For this review, take the finished solid that the model builds, in its own axes (mm). A direction names the side the tool comes from. Give positions to 0.01 mm unless a question says otherwise; leave off trailing zeros. Write each loop counter-clockwise with the first axis right and the second up, starting at its lowest first coordinate (ties: lowest second). Pieces come first, ordered by that corner, then holes. Notation, with made-up numbers: M 85,-30.5 L 96,-30.5 A26 cw 96,-5.5 Z; hole C 85,2 d5. An arc over 180 degrees is marked long. Use one line per item in the form item = value. Start each with the question number.
Q1. Clearance check with flat-ended pins moving along their axes: pin 1 Ø1.8 at (y, z) = (5.5, 4) entering from +X; pin 2 Ø1.7 at (x, y) = (8, -3) entering from -Z; pin 3 Ø2.5 at (y, z) = (5, 8.5) entering from -X; pin 4 Ø4 at (x, z) = (0, 0) entering from -Y. State where each tip first meets the part, or that it passes through.
Q2. Consider section A-A on x = -82.55. Write out the cut boundary in (y, z).
Q3. Consider section C-C on x = -16. Write out the cut boundary in (y, z), and give its area (3 significant figures).
Q4. Tool access review of faces 1 (the flat face through (0, -3, -4.158)), 2 (the flat face through (-83, 4, 4.158)), 3 (the flat face through (-154, -16, 0.211)), 4 (the flat face through (-42, -3, -10)): name each direction out of +Z, -Z, +X, -X, +Y, -Y from which nothing blocks a thin tool from reaching the whole face with its end or side.
Q5. Mouldability with a two-part tool opening along Z and no side actions: class faces 5 (the cylindrical face through (-145.455, -23.522, -2.686)), 6 (the flat face through (-74, -6.35, 0)), 7 (the cylindrical face through (-85.967, -1.878, -0.759)) as released by +Z, released by -Z, zero draft, split by the parting line, or undercut.
Q6. For probe 1 along X at (y, z) = (-1, 0); probe 2 along X at (y, z) = (-2, -2.5); probe 3 along Y at (x, z) = (-106, 3.5), list the stretches that pass through material, from the lowest coordinate up. Write a range as [from, to].
Q7. Consider section B-B on y = -21.5. Write out the cut boundary in (x, z).
Q8. Consider section D-D on z = -6. Give the number of separate pieces and of enclosed holes in the cut face, and give its area (3 significant figures).
```python
from build123d import *

# Parameters (mm, degrees)
BOSS_EXTRUDE1_DEPTH   = 7.62
BOSS_EXTRUDE1_2_DEPTH = 7.62
BOSS_EXTRUDE1_3_DEPTH = 7.62
BOSS_EXTRUDE1_4_DEPTH = 7.62
SKETCH2_W             = 165.1
SKETCH2_H             = 20
BOSS_EXTRUDE2_DEPTH   = 6.35
LPATTERN2_COUNT       = 2
LPATTERN2_PITCH       = 82.55
CUT_EXTRUDE1_DEPTH    = 157.048617104
FILLET1_R             = 2.54
SKETCH13_R            = 3.5
CUT_EXTRUDE5_DEPTH    = 156.608722121
FILLET6_R             = 2.54
SKETCH14_W            = 8.89
SKETCH14_H            = 5.842
CUT_EXTRUDE6_DEPTH    = 157.048617104
SKETCH15_W            = 25.4
SKETCH15_H            = 40.894
BOSS_EXTRUDE3_DEPTH   = 12.7
FILLET15_R            = 10.16
FILLET16_R            = 10.16
FILLET17_R            = 10.16
FILLET18_R            = 10.16
SKETCH18_R            = 1.984375
CUT_EXTRUDE9_DEPTH    = 12.7


with BuildPart() as part:
    # Sketch1 → Boss-Extrude1 (new body)
    with BuildSketch(Plane(origin=(0, 0, 0), x_dir=(1, 0, 0), z_dir=(0, 1, 0))):
        Polygon((2.9718, 10), (-2.9718, 10), (-2.9718, 7.714), (-4.567901235, 7.714), (-4.567901235, 6.444), (-2.9718, 4.158), (2.9718, 4.158), (4.322098765, 6.444), (4.322098765, 7.714), (2.9718, 7.714), align=None)
    boss_extrude1 = extrude(amount=BOSS_EXTRUDE1_DEPTH)



with BuildPart() as body_2:
    # Sketch1 → Boss-Extrude1 2 (new body)
    with BuildSketch(Plane(origin=(0, 0, 0), x_dir=(1, 0, 0), z_dir=(0, 1, 0))):
        Polygon((4.158, -2.9718), (4.158, 2.9718), (6.444, 4.322098765), (7.714, 4.322098765), (7.714, 2.9718), (10, 2.9718), (10, -2.9718), (7.714, -2.9718), (7.714, -4.567901235), (6.444, -4.567901235), align=None)
    boss_extrude1_2 = extrude(amount=BOSS_EXTRUDE1_2_DEPTH)


with BuildPart() as body_3:
    # Sketch1 → Boss-Extrude1 3 (new body)
    with BuildSketch(Plane(origin=(0, 0, 0), x_dir=(1, 0, 0), z_dir=(0, 1, 0))):
        Polygon((-10, -2.9718), (-10, 2.9718), (-7.714, 2.9718), (-7.714, 4.567901235), (-6.444, 4.567901235), (-4.158, 2.9718), (-4.158, -2.9718), (-6.444, -4.322098765), (-7.714, -4.322098765), (-7.714, -2.9718), align=None)
    boss_extrude1_3 = extrude(amount=BOSS_EXTRUDE1_3_DEPTH)


with BuildPart() as body_4:
    # Sketch1 → Boss-Extrude1 4 (new body)
    with BuildSketch(Plane(origin=(0, 0, 0), x_dir=(1, 0, 0), z_dir=(0, 1, 0))):
        Polygon((4.567901235, -6.444), (2.9718, -4.158), (-2.9718, -4.158), (-4.322098765, -6.444), (-4.322098765, -7.714), (-2.9718, -7.714), (-2.9718, -10), (2.9718, -10), (2.9718, -7.714), (4.567901235, -7.714), align=None)
    boss_extrude1_4 = extrude(amount=BOSS_EXTRUDE1_4_DEPTH)


with BuildPart() as part_1:
    add(part.part)

    add(body_2.part)  # Boss-Extrude2 merges body 2

    add(body_3.part)  # Boss-Extrude2 merges body 3

    add(body_4.part)  # Boss-Extrude2 merges body 4
    # Sketch2 → Boss-Extrude2 (add)
    with BuildSketch(Plane.XZ):
        with Locations((-72.55, 0)):
            Rectangle(SKETCH2_W, SKETCH2_H)
    extrude(amount=BOSS_EXTRUDE2_DEPTH)

    # LPattern2: Boss-Extrude1, Boss-Extrude1 2, Boss-Extrude1 3, Boss-Extrude1 4 ×2
    with Locations(*[(-i * LPATTERN2_PITCH, 0, 0) for i in range(1, LPATTERN2_COUNT)]):
        add(boss_extrude1)
        add(boss_extrude1_2)
        add(boss_extrude1_3)
        add(boss_extrude1_4)

    # Sketch4 → Cut-Extrude1 (cut, through all)
    with BuildSketch(Plane(origin=(0, -6.35, 0), x_dir=(-1, 0, 0), z_dir=(0, -1, 0))):
        Polygon((155.1, -10), (117.5588, -10), (155.1, -0.2108), align=None)
    extrude(amount=-CUT_EXTRUDE1_DEPTH, mode=Mode.SUBTRACT)

    # Fillet1
    fillet1_edges = [part_1.edges().sort_by_distance(p)[0] for p in [
        (-117.5588, -3.175, 10),
    ]]
    fillet(fillet1_edges, radius=FILLET1_R)

    # Sketch13 → Cut-Extrude5 (cut, through all)
    with BuildSketch(Plane(origin=(0, 0, 0), x_dir=(1, 0, 0), z_dir=(0, 1, 0))):
        with Locations(Location((0, 0, 0), (0, 0, 270))):
            Circle(SKETCH13_R)
        with Locations(Location((-82.55, 0, 0), (0, 0, 270))):
            Circle(SKETCH13_R)
    extrude(amount=-CUT_EXTRUDE5_DEPTH, mode=Mode.SUBTRACT)

    # Fillet6
    fillet6_edges = [part_1.edges().sort_by_distance(p)[0] for p in [
        (0, -6.35, -3.5),
        (-82.55, -6.35, -3.5),
    ]]
    fillet(fillet6_edges, radius=FILLET6_R)

    # Sketch14 → Cut-Extrude6 (cut, through all)
    with BuildSketch(Plane(origin=(0, 7.62, 0), x_dir=(1, 0, 0), z_dir=(0, 1, 0))):
        with Locations((-0.122901235, 7.079)):
            Rectangle(SKETCH14_W, SKETCH14_H)
        with Locations((-82.672901235, 7.079)):
            Rectangle(SKETCH14_W, SKETCH14_H)
    extrude(amount=-CUT_EXTRUDE6_DEPTH, mode=Mode.SUBTRACT)

    # Sketch15 → Boss-Extrude3 (add)
    with BuildSketch(Plane.ZY.offset(155.1)):
        with Locations((-12.4892, -20.447)):
            Rectangle(SKETCH15_W, SKETCH15_H)
    extrude(amount=-BOSS_EXTRUDE3_DEPTH)

    # Fillet15
    fillet15_edges = [part_1.edges().sort_by_distance(p)[0] for p in [
        (-142.4, -6.35, -4.8946),
    ]]
    fillet(fillet15_edges, radius=FILLET15_R)

    # Fillet16
    fillet16_edges = [part_1.edges().sort_by_distance(p)[0] for p in [
        (-142.4, -8.255, -10),
    ]]
    fillet(fillet16_edges, radius=FILLET16_R)

    # Fillet17
    fillet17_edges = [part_1.edges().sort_by_distance(p)[0] for p in [
        (-142.4, -40.894, -12.4892),
    ]]
    fillet(fillet17_edges, radius=FILLET17_R)

    # Fillet18
    fillet18_edges = [part_1.edges().sort_by_distance(p)[0] for p in [
        (-139.424204897, -9.325795103, 0.2108),
        (-153.83, -40.894, 0.2108),
        (-142.4, -23.622, 0.2108),
        (-145.375795103, -37.918204897, 0.2108),
    ]]
    fillet(fillet18_edges, radius=FILLET18_R)

    # Sketch18 → Cut-Extrude9 (cut)
    with BuildSketch(Plane.ZY.offset(155.1)):
        with Locations((-12.4892, -28.194)):
            Circle(SKETCH18_R)
    extrude(amount=-CUT_EXTRUDE9_DEPTH, mode=Mode.SUBTRACT)


solid = part_1.part
```
Working result:
q1.pin_1 = 7.71
q1.pin_2 = -10
q1.pin_3 = -86.87
q1.pin_4 = through
q2.outline = M -6.35,6.04 A2.54 ccw -3.81,3.5 L 0,3.5 L 0,4.16 L 7.62,4.16 L 7.62,10 L -6.35,10 Z; M -5.52,-4.16 L 0,-4.16 L 0,-3.5 L -3.81,-3.5 A2.54 ccw Z
q3.outline = M -6.35,-10 L 0,-10 L 0,10 L -6.35,10 Z
q3.area = 127 mm²
q4.face_1 = -Z, +Y, -Y
q4.face_2 = -Z, +Y
q4.face_3 = +Z, +X, -X, -Y
q4.face_4 = -Z, +X, +Y, -Y
q5.face_5 = released by +Z
q5.face_6 = zero draft
q5.face_7 = undercut
q6.probe_1 = [-155.1, -86.05], [-79.05, -3.5], [3.5, 10]
q6.probe_2 = [-155.1, -85], [-80.1, -2.45], [2.45, 10]
q6.probe_3 = [-6.35, 0]
q7.outline = M -155.1,-25.19 L -142.4,-25.19 L -142.4,-9.95 A10.16 ccw -152.56,0.21 L -155.1,0.21 Z
q8.separate_pieces = 3
q8.enclosed_holes = 0
q8.area = 1,340 mm²
